Source: CAD feature listing. Evaluate the final solid. Frame: model axes, mm. Round coordinates to 2 decimals unless told otherwise and drop trailing zeros. Loops run counter-clockwise (first coordinate to the right, second up) from the corner with the lowest first, then second, coordinate; pieces in that order, holes last. Notation, with made-up numbers: (15.25, -25) -> (70.25, -25) arc R16 cw to (70.25, -17) -> close; hole circle Ø6 at (7, -28). An arc over 180 degrees is marked (long way). Write item = value, one per line.
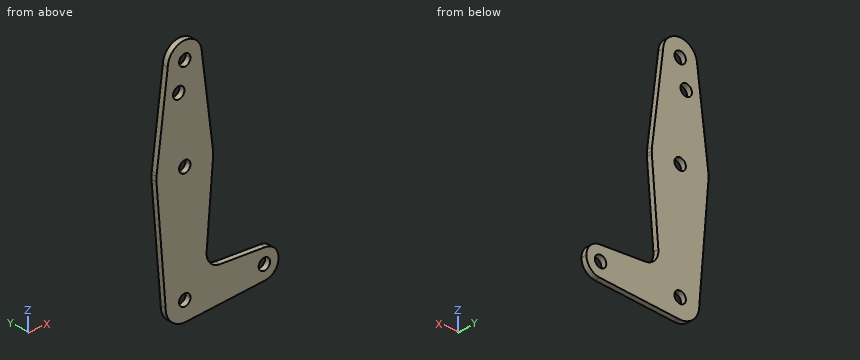
from build123d import *

# Parameters (mm, degrees)
F0_R     = 3.175
F1_DEPTH = 3.048


# Not quite as in the source:
# - ends of sketch curves that miss each other by under 0.0002 mm in the source are joined


with BuildPart() as f1:
    # F0 (on Front) → F1 (new body)
    with BuildSketch(Plane.XZ):
        with BuildLine():
            ThreePointArc((0, -42.9560914541), (7.5600620245, -46.0875716771), (10.6915422474, -53.6476337016))
            Line((10.6915422474, -53.6476337016), (36.5125, -53.6476337016))
            ThreePointArc((36.5125, -53.6476337016), (39.0126759444, -47.8649515069), (44.9381789581, -45.725160126))
            Line((44.9381789581, -45.725160126), (19.6163710563, -44.1648504083))
            ThreePointArc((19.6163710563, -44.1648504083), (14.0942781367, -41.4328681595), (12.1820328049, -35.5762005907))
            Line((12.1820328049, -35.5762005907), (15.8212777121, 8.5474538872))
            ThreePointArc((15.8212777121, 8.5474538872), (10.7540722598, -1.825200003), (0, -6.0226337016))
            Line((0, -6.0226337016), (0, -42.9560914541))
        make_face()
        with BuildLine():
            ThreePointArc((-10.690047341, -53.4688503814), (-7.4965860966, -46.0246242876), (0, -42.9560914541))
            Line((0, -42.9560914541), (0, -6.0226337016))
            ThreePointArc((0, -6.0226337016), (-10.7540722823, -1.8251999914), (-15.8212777256, 8.5474539313))
            Line((-15.8212777256, 8.5474539313), (-10.690047341, -53.4688503814))
        make_face()
        with BuildLine():
            Line((10.6915422474, -53.6476337016), (3.175, -53.6476337016))
            ThreePointArc((3.175, -53.6476337016), (-2.2450640303, -55.8926977318), (0, -50.4726337016))
            Line((0, -50.4726337016), (0, -42.9560914541))
            ThreePointArc((0, -42.9560914541), (-7.4965860966, -46.0246242876), (-10.690047341, -53.4688503814))
            ThreePointArc((-10.690047341, -53.4688503814), (-7.6230094139, -61.1442197982), (0, -64.339175949))
            Line((0, -64.339175949), (1.3126312246, -64.2582922531))
            ThreePointArc((1.3126312246, -64.2582922531), (8.0107155679, -60.7284183839), (10.6915422474, -53.6476337016))
        make_face()
        with BuildLine():
            ThreePointArc((0, -50.4726337016), (2.2450640303, -51.4025696713), (3.175, -53.6476337016))
            Line((3.175, -53.6476337016), (10.6915422474, -53.6476337016))
            ThreePointArc((10.6915422474, -53.6476337016), (7.5600620245, -46.0875716771), (0, -42.9560914541))
            Line((0, -42.9560914541), (0, -50.4726337016))
        make_face()
        with BuildLine():
            Line((36.5125, -53.6476337016), (10.6915422474, -53.6476337016))
            ThreePointArc((10.6915422474, -53.6476337016), (8.0107155679, -60.7284183839), (1.3126312246, -64.2582922531))
            Line((1.3126312246, -64.2582922531), (44.9381789581, -61.5701072771))
            ThreePointArc((44.9381789581, -61.5701072771), (39.0126759444, -59.4303158963), (36.5125, -53.6476337016))
        make_face()
        with BuildLine():
            ThreePointArc((44.9381789581, -45.725160126), (39.0126759444, -47.8649515069), (36.5125, -53.6476337016))
            ThreePointArc((36.5125, -53.6476337016), (39.0126759444, -59.4303158963), (44.9381789581, -61.5701072771))
            ThreePointArc((44.9381789581, -61.5701072771), (50.2326821947, -59.0849577571), (52.3875, -53.6476337016))
            ThreePointArc((52.3875, -53.6476337016), (50.2326821947, -48.210309646), (44.9381789581, -45.725160126))
        make_face()
        with BuildLine():
            ThreePointArc((47.625, -53.6476337016), (44.45, -56.8226337016), (41.275, -53.6476337016))
            ThreePointArc((41.275, -53.6476337016), (44.45, -50.4726337016), (47.625, -53.6476337016))
        make_face(mode=Mode.SUBTRACT)
        with BuildLine():
            ThreePointArc((-15.8212777256, 8.5474539313), (-10.7540722823, -1.8251999914), (0, -6.0226337016))
            Line((0, -6.0226337016), (0, 6.6773662984))
            ThreePointArc((0, 6.6773662984), (-3.1750000049, 9.8523662984), (0, 13.0273662984))
            Line((0, 13.0273662984), (0, 25.7273662984))
            ThreePointArc((0, 25.7273662984), (-10.2345652868, 21.9878225524), (-15.6473851089, 12.5309787019))
            Line((-15.6473851089, 12.5309787019), (-15.8212782601, 11.157272185))
            ThreePointArc((-15.8212782601, 11.157272185), (-15.8750000049, 9.8523630471), (-15.8212777256, 8.5474539313))
        make_face()
        with BuildLine():
            Line((0, 6.6773662984), (0, -6.0226337016))
            ThreePointArc((0, -6.0226337016), (10.7540722598, -1.825200003), (15.8212777121, 8.5474538872))
            ThreePointArc((15.8212777121, 8.5474538872), (15.8615637383, 9.1993574002), (15.8749999951, 9.8523662984))
            ThreePointArc((15.8749999951, 9.8523662984), (15.843418635, 10.8532213331), (15.7488002092, 11.8500942118))
            ThreePointArc((15.7488002092, 11.8500942118), (10.4952773724, 21.7630664363), (0, 25.7273662984))
            Line((0, 25.7273662984), (0, 13.0273662984))
            ThreePointArc((0, 13.0273662984), (2.2450640271, 12.097430327), (3.1749999951, 9.8523662984))
            ThreePointArc((3.1749999951, 9.8523662984), (2.2450640271, 7.6073022699), (0, 6.6773662984))
        make_face()
        with BuildLine():
            ThreePointArc((0, 25.7273662984), (10.4952773724, 21.7630664363), (15.7488002092, 11.8500942118))
            Line((15.7488002092, 11.8500942118), (9.5202989573, 60.9515865588))
            ThreePointArc((9.5202989573, 60.9515865588), (9.5238246668, 60.801994892), (9.525, 60.6523662984))
            ThreePointArc((9.525, 60.6523662984), (6.7351920908, 53.9171742076), (0, 51.1273662984))
            Line((0, 51.1273662984), (0, 25.7273662984))
        make_face()
        with BuildLine():
            Line((-9.5210262398, 60.9274741696), (-15.6473851089, 12.5309787019))
            ThreePointArc((-15.6473851089, 12.5309787019), (-10.2345652868, 21.9878225524), (0, 25.7273662984))
            Line((0, 25.7273662984), (0, 51.1273662984))
            ThreePointArc((0, 51.1273662984), (-6.8317650528, 54.0151521793), (-9.5210262398, 60.9274741696))
        make_face()
        with Locations((-3.3664405459, 46.3775662984)):
            Circle(F0_R, mode=Mode.SUBTRACT)
        with BuildLine():
            ThreePointArc((9.5202989573, 60.9515865588), (-0.0120616774, 70.1773586615), (-9.5210262398, 60.9274741696))
            ThreePointArc((-9.5210262398, 60.9274741696), (-6.8317650528, 54.0151521793), (0, 51.1273662984))
            ThreePointArc((0, 51.1273662984), (6.7351920908, 53.9171742076), (9.525, 60.6523662984))
            ThreePointArc((9.525, 60.6523662984), (9.5238246668, 60.801994892), (9.5202989573, 60.9515865588))
        make_face()
        with BuildLine():
            ThreePointArc((3.175, 60.6523662984), (2.2450640303, 58.4073022682), (0, 57.4773662984))
            ThreePointArc((0, 57.4773662984), (-2.2450640303, 62.8974303287), (3.175, 60.6523662984))
        make_face(mode=Mode.SUBTRACT)
    extrude(amount=F1_DEPTH)


solid = f1.part
1. Contact query for flat-ended pins moving along their axis: pin 1 Ø1 at (y, z) = (-1.5, 10) entering from +X (3 decimals); pin 2 Ø1.5 at (y, z) = (-0.5, 32.5) entering from +X. Output: stop coordinate, or through.
Evaluation:
pin_1 = 15.875
pin_2 = 13.22
2. Section query A-A (x = -4.5). Return the cut outline in (y, z), then the cut area to 3 significant figures.
Evaluation:
outline = (-3.05, -63.35) -> (0, -63.35) -> (0, 43.41) -> (-3.05, 43.41) -> close; (-3.05, 49.34) -> (0, 49.34) -> (0, 69.05) -> (-3.05, 69.05) -> close
area = 385 mm²
3. Section query B-B (y = -1.45). Give the number of separate pieces and of enclosed holes in the cut face, then the cut area to 3 significant figures.
Evaluation:
separate_pieces = 1
enclosed_holes = 5
area = 3,890 mm²
4. Line query: probe 1 along Z at (x, y) = (44.45, -1.3); probe 2 along X at (y, z) = (-2.6, 59); probe 3 along X at (y, z) = (-1.6, 7). Output: solid intervals per line, ascending. Write a range as from..to.
Evaluation:
probe_1 = -61.6..-56.82, -50.47..-45.7
probe_2 = -9.77..-2.71, 2.71..9.77
probe_3 = -15.69..-1.39, 1.39..15.69
5. Section query D-D (z = -2.5). Return the cut outline in (x, y), then the cut area to 3 significant figures.
Evaluation:
outline = (-14.91, -3.05) -> (14.91, -3.05) -> (14.91, 0) -> (-14.91, 0) -> close
area = 90.9 mm²
6. Section query C-C (z = 35.5). Return the cut outline in (x, y).
Evaluation:
outline = (-12.74, -3.05) -> (12.75, -3.05) -> (12.75, 0) -> (-12.74, 0) -> close
